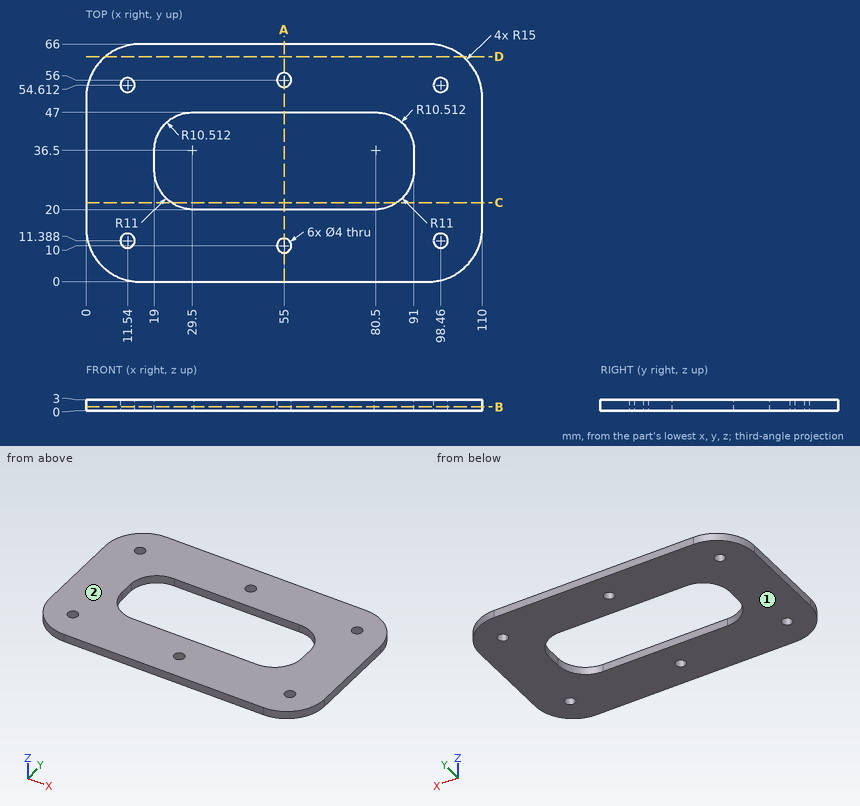
The figure shows three views and two pictorial views of one solid part (mm, origin at its lowest corner). Answer the questions. Give positions to 0.01 mm unless a question says otherwise; leave off trailing zeros. Write each loop counter-clockwise with the first axis right and the second up, starting at its lowest first coordinate (ties: lowest second). Pieces come first, ordered by that corner, then holes.
Q1. The part is cut by section C-C on y = 22. Give the vertices of the cut face in (x, z) (1 decimal), and give its area (3 significant figures).
Answer:
outline: (0, 0) - (23.7, 0) - (23.7, 3) - (0, 3) - close; (86.3, 0) - (110, 0) - (110, 3) - (86.3, 3) - close
area: 142 mm2
Q2. Given pin 1 (4.5 mm diameter, centred on x = 98.46, y = 11.39, fed in from -Z); pin 2 (3.5 mm diameter, centred on x = 55, y = 56, fed in from -Z), each flat-ended and moving along its own axis, determine where each tip first touches the part or whether it passes through.
Answer:
pin 1: stops at z = 0
pin 2: passes through
Q3. The part is cut by section D-D on y = 62.5. Give the vertices of the cut face in (x, z).
Answer:
outline: (5.37, 0) - (104.63, 0) - (104.63, 3) - (5.37, 3) - close
Q4. Straight lines are drawn through the part: L1, parallel to Y at x = 55, z = 0.8; L2, parallel to Y at x = 68, z = 2.15; L3, parallel to Y at x = 11.5, z = 1.8 (1 decimal). For each, find the intervals that lie inside material, in ascending order.
Answer:
L1: y = 0 to 8, 12 to 20, 47 to 54, 58 to 66
L2: y = 0 to 20, 47 to 66
L3: y = 0.4 to 9.4, 13.4 to 52.6, 56.6 to 65.6
Q5. The part is cut by section A-A on x = 55. Give the vertices of the cut face in (y, z).
Answer:
outline: (0, 0) - (8, 0) - (8, 3) - (0, 3) - close; (12, 0) - (20, 0) - (20, 3) - (12, 3) - close; (47, 0) - (54, 0) - (54, 3) - (47, 3) - close; (58, 0) - (66, 0) - (66, 3) - (58, 3) - close
Q6. The part is cut by section B-B on z = 1.05. Give the vertices of the cut face in (x, y).
Answer:
outline: (0, 15) arc R15 ccw to (15, 0) - (95, 0) arc R15 ccw to (110, 15) - (110, 51) arc R15 ccw to (95, 66) - (15, 66) arc R15 ccw to (0, 51) - close; hole circle Ø4 at (11.54, 11.39); hole circle Ø4 at (11.54, 54.61); hole (19, 31) arc R11 ccw to (30, 20) - (80, 20) arc R11 ccw to (91, 31) - (91, 37) arc R10.51 ccw to (80, 47) - (30, 47) arc R10.51 ccw to (19, 37) - close; hole circle Ø4 at (55, 10); hole circle Ø4 at (55, 56); hole circle Ø4 at (98.46, 11.39); hole circle Ø4 at (98.46, 54.61)
Q7. For a pull along Z with two mould halves and no side action, classify the marked faces 1 and 2 as released by +Z, released by -Z, zero draft, split by the parting line, or undercut.
Answer:
face 1: released by -Z
face 2: released by +Z
